Geometry check sheet. Reference: the model listing, model coordinates, mm. A direction names the side the tool comes from. Round coordinates to 2 decimals unless told otherwise and drop trailing zeros. Order: outer loops, then holes, each group sorted by start corner. A loop starts at its lowest first (then second) coordinate and runs counter-clockwise, first axis right, second up. Notation, with made-up numbers: (-2.75, -21) - (13.25, -21) arc R36 ccw to (13.25, 14) - close; hole circle Ø11 at (86, 46.5). An arc over 180 degrees is marked (long way). Answer as CSV lines item,"result". Start each with the question number.
```python
from build123d import *

# Parameters (mm, degrees)
BOSS_EXTRUDE1_DEPTH   = 1
BOSS_EXTRUDE1_2_DEPTH = 1
BOSS_EXTRUDE2_DEPTH   = 3
SKETCH1_4_R           = 0.5
BOSS_EXTRUDE3_DEPTH   = 2.5


with BuildPart() as part:
    # Sketch1 → Boss-Extrude1 (new body)
    with BuildSketch(Plane(origin=(0, 0, 0), x_dir=(1, 0, 0), z_dir=(0, 1, 0))):
        with BuildLine():
            ThreePointArc((3.5, 1), (2.5, 0), (3.5, -1))
            Line((3.5, -1), (3.5, 1))
        make_face()
    extrude(amount=BOSS_EXTRUDE1_DEPTH)



with BuildPart() as body_2:
    # Sketch1 → Boss-Extrude1 2 (new body)
    with BuildSketch(Plane(origin=(0, 0, 0), x_dir=(1, 0, 0), z_dir=(0, 1, 0))):
        with BuildLine():
            Line((-3.5, 1), (-3.5, -1))
            ThreePointArc((-3.5, -1), (-2.792893219, -0.707106781), (-2.5, 0))
            ThreePointArc((-2.5, 0), (-2.792893219, 0.707106781), (-3.5, 1))
        make_face()
    extrude(amount=BOSS_EXTRUDE1_2_DEPTH)


with BuildPart() as part_1:
    add(part.part)

    add(body_2.part)  # Boss-Extrude2 merges body 2
    # Sketch1_3 → Boss-Extrude2 (add)
    with BuildSketch(Plane(origin=(0, 0, 0), x_dir=(1, 0, 0), z_dir=(0, 1, 0))):
        with BuildLine():
            Line((-3.5, -2), (0, -2))
            Line((0, -2), (-2, 2))
            Line((-2, 2), (-3.5, 2))
            Line((-3.5, 2), (-3.5, 1))
            ThreePointArc((-3.5, 1), (-2.792893219, 0.707106781), (-2.5, 0))
            ThreePointArc((-2.5, 0), (-2.792893219, -0.707106781), (-3.5, -1))
            Line((-3.5, -1), (-3.5, -2))
        make_face()
        with BuildLine():
            Line((0, 2), (2, -2))
            Line((2, -2), (3.5, -2))
            Line((3.5, -2), (3.5, -1))
            ThreePointArc((3.5, -1), (2.5, 0), (3.5, 1))
            Line((3.5, 1), (3.5, 2))
            Line((3.5, 2), (0, 2))
        make_face()
    extrude(amount=BOSS_EXTRUDE2_DEPTH)

    # Sketch1_4 → Boss-Extrude3 (add)
    with BuildSketch(Plane(origin=(0, 0, 0), x_dir=(1, 0, 0), z_dir=(0, 1, 0))):
        Polygon((-2, 2), (0, -2), (2, -2), (0, 2), align=None)
        Circle(SKETCH1_4_R, mode=Mode.SUBTRACT)
    extrude(amount=BOSS_EXTRUDE3_DEPTH)


solid = part_1.part
```
1. Section check D-D on x = -1. Record the boundary of the cut face in (y, z), plus the area to 3 significant figures.
2. Section check C-C on x = -0.25. Record the boundary of the cut face in (y, z).
3. Thickness scan on probe 1 along X at (y, z) = (1.3, 0); probe 2 along Z at (x, y) = (0, 1.95); probe 3 along Y at (x, z) = (0.25, 1.7). Record the ranges inside material, lowest first.
4. Section check A-A on y = 1.2. Record the boundary of the cut face in (x, z), plus the area to 3 significant figures.
5. Access from +Z, -Z, +X, -X, +Y, -Y to the whole of each face (thin tool, end or side, straight path). Record for faces 1 (the face through (-2, 3, 0)), 2 (the face through (-0.5, 2.5, -0.5)), 3 (the face through (-3.5, 0.8, 0)), 4 (the face through (-1, 2.7, 0)), 5 (the face through (3, 1, 0)).
6. Draft check along X on faces 6 (the face through (-3, 1, 0)), 7 (the face through (1, 2.7, 0)), 8 (the face through (2.5, 2, 0)). Enter one of: released by +X, released by -X, zero draft, split by the parting line, or undercut.
7. Section check B-B on z = -0.8. Record the boundary of the cut face in (x, y), plus the area to 3 significant figures.
Numbers:
1,outline,"(0, -2) - (2.5, -2) - (2.5, 0) - (3, 0) - (3, 2) - (0, 2) - close"
1,area,"11.0 mm2"
2,outline,"(0, -2) - (2.5, -2) - (2.5, -0.43) - (0, -0.43) - close; (0, 0.43) - (2.5, 0.43) - (2.5, 1.5) - (3, 1.5) - (3, 2) - (0, 2) - close"
3,probe 1,"x = -2.5 to -0.5, 0.5 to 2.5"
3,probe 2,"z = -2 to -0.5, 0.5 to 2"
3,probe 3,"y = 0 to 2.5"
4,outline,"(-3.5, -2) - (3.5, -2) - (3.5, -1) arc R1 cw to (3.5, 1) - (3.5, 2) - (-3.5, 2) - (-3.5, 1) arc R1 cw to (-3.5, -1) - close; hole circle Ø1 at (0, 0)"
4,area,"24.1 mm2"
5,face 1,"+Z, -Z, +X, -X, +Y"
5,face 2,"+Y"
5,face 3,"+Z, -Z, -X, +Y, -Y"
5,face 4,"-Z, +Y"
5,face 5,"+X, +Y"
6,face 6,"zero draft"
6,face 7,"undercut"
6,face 8,"released by +X"
7,outline,"(-3.5, 0) - (3.5, 0) - (3.5, 1) - (2.9, 1) - (2.9, 3) - (0.6, 3) - (0.6, 2.5) - (-1.4, 2.5) - (-1.4, 3) - (-2.9, 3) - (-2.9, 1) - (-3.5, 1) - close"
7,area,"17.6 mm2"
